Can you work these out from the model? Positions are in its coordinate system, mm. A direction names the side the tool comes from. Give positions to 0.01 mm unless a question says otherwise; leave off trailing zeros. Loops run counter-clockwise (first coordinate to the right, second up) from the corner with the lowest first, then second, coordinate; pieces in that order, holes last. Notation, with made-up numbers: (71.5, 23) -> (122.5, 23) arc R21 cw to (122.5, 37) -> close; hole circle Ø9 at (62, 67.5). An arc over 180 degrees is marked (long way). One line per question, with ' | ' between items.
from build123d import *

# Parameters (mm, degrees)
BOSS_EXTRUDE1_DEPTH      = 5
CHASSIS_WALLS1_DEPTH     = 12
CHAMFER1_SIZE            = 10
CHAMFER2_SIZE            = 10
CHAMFER3_SIZE            = 2.5
SKETCH4_R                = 1.65
CUT_EXTRUDE1_DEPTH       = 10
SKETCH5_W                = 55
SKETCH5_H                = 11
CUT_EXTRUDE2_DEPTH       = 10
SKETCH6_W                = 65
SKETCH6_H                = 5
CUT_EXTRUDE3_DEPTH       = 6
FILLET1_R                = 10
SKETCH7_W                = 42.9
SKETCH7_H                = 22
CUT_EXTRUDE4_DEPTH       = 6
SKETCH9_R                = 1.625
CUT_EXTRUDE5_DEPTH       = 6
SKETCH10_W               = 10
SKETCH10_H               = 13
SERVO_CABLE_CUTOUT_DEPTH = 10
FILLET2_R                = 2
SKETCH11_R               = 1.6
CUT_EXTRUDE6_DEPTH       = 6


with BuildPart() as part:
    # Sketch1 → Boss-Extrude1 (new body)
    with BuildSketch(Plane(origin=(0, 0, 0), x_dir=(1, 0, 0), z_dir=(0, 1, 0))):
        Polygon((-95, 35), (-65, 55), (65, 55), (95, 30), (170, 30), (170, -30), (95, -30), (65, -55), (-65, -55), (-95, -35), (-155, -35), (-155, 35), align=None)
    extrude(amount=BOSS_EXTRUDE1_DEPTH)

    # Sketch3 → Chassis-Walls1 (add)
    with BuildSketch(Plane(origin=(0, 5, 0), x_dir=(1, 0, 0), z_dir=(0, 1, 0))):
        Polygon((0, 55), (-65, 55), (-95, 35), (-92.226499019, 30.839748528), (-62.226499019, 50.839748528), (0, 50.839748528), (61.533123774, 50.839748528), (83.850910978, 32.241592525), (87.317787204, 36.401843997), (65, 55), align=None)
        Polygon((61.533123774, -50.839748528), (0, -50.839748528), (-62.226499019, -50.839748528), (-92.226499019, -30.839748528), (-95, -35), (-65, -55), (0, -55), (65, -55), (87.317787204, -36.401843997), (83.850910978, -32.241592525), align=None)
    extrude(amount=CHASSIS_WALLS1_DEPTH)

    # Chamfer1
    chamfer1_edges = [part.edges().sort_by_distance(p)[0] for p in [
        (-155, 2.5, 35),
        (-155, 2.5, -35),
    ]]
    chamfer(chamfer1_edges, length=CHAMFER1_SIZE)

    # Chamfer2
    chamfer2_edges = [part.edges().sort_by_distance(p)[0] for p in [
        (170, 2.5, -30),
        (170, 2.5, 30),
    ]]
    chamfer(chamfer2_edges, length=CHAMFER2_SIZE)

    # Chamfer3
    chamfer3_edges = [part.edges().sort_by_distance(p)[0] for p in [
        (-93.613249509, 17, -32.919874264),
        (85.584349091, 17, -34.321718261),
        (-93.613249509, 17, 32.919874264),
        (85.584349091, 17, 34.321718261),
    ]]
    chamfer(chamfer3_edges, length=CHAMFER3_SIZE)

    # Sketch4 → Cut-Extrude1 (cut)
    with BuildSketch(Plane.XZ):
        with Locations((-147, 17)):
            Circle(SKETCH4_R)
        with Locations((-55, 17)):
            Circle(SKETCH4_R)
        with Locations((-55, -17)):
            Circle(SKETCH4_R)
        with Locations((-147, -17)):
            Circle(SKETCH4_R)
        with Locations((-25, 31)):
            Circle(SKETCH4_R)
        with Locations((60, 31)):
            Circle(SKETCH4_R)
        with Locations((60, -31)):
            Circle(SKETCH4_R)
        with Locations((-25, -31)):
            Circle(SKETCH4_R)
    extrude(amount=-CUT_EXTRUDE1_DEPTH, mode=Mode.SUBTRACT)

    # Sketch5 → Cut-Extrude2 (cut)
    with BuildSketch(Plane(origin=(0, 5, 0), x_dir=(1, 0, 0), z_dir=(0, 1, 0))):
        with Locations((-127.5, -29.5)):
            Rectangle(SKETCH5_W, SKETCH5_H)
    extrude(amount=-CUT_EXTRUDE2_DEPTH, mode=Mode.SUBTRACT)

    # Sketch6 → Cut-Extrude3 (cut, through all)
    with BuildSketch(Plane(origin=(0, 5, 0), x_dir=(1, 0, 0), z_dir=(0, 1, 0))):
        with Locations((17.5, 22.5)):
            Rectangle(SKETCH6_W, SKETCH6_H)
        with Locations((17.5, -22.5)):
            Rectangle(SKETCH6_W, SKETCH6_H)
    extrude(amount=-CUT_EXTRUDE3_DEPTH, mode=Mode.SUBTRACT)

    # Fillet1
    fillet1_edges = [part.edges().sort_by_distance(p)[0] for p in [
        (-100, 2.5, 24),
    ]]
    fillet(fillet1_edges, radius=FILLET1_R)

    # Sketch7 → Cut-Extrude4 (cut, through all)
    with BuildSketch(Plane(origin=(0, 5, 0), x_dir=(1, 0, 0), z_dir=(0, 1, 0))):
        with Locations((141.25, 0)):
            Rectangle(SKETCH7_W, SKETCH7_H)
    extrude(amount=-CUT_EXTRUDE4_DEPTH, mode=Mode.SUBTRACT)

    # Sketch9 → Cut-Extrude5 (cut, through all)
    with BuildSketch(Plane(origin=(0, 5, 0), x_dir=(1, 0, 0), z_dir=(0, 1, 0))):
        with Locations((117, -19)):
            Circle(SKETCH9_R)
        with Locations((145, -19)):
            Circle(SKETCH9_R)
        with Locations((162, -17)):
            Circle(SKETCH9_R)
    cut_extrude5 = extrude(amount=-CUT_EXTRUDE5_DEPTH, mode=Mode.SUBTRACT)

    # Mirror1: Cut-Extrude5 across plane
    add(cut_extrude5.mirror(Plane.XY), mode=Mode.SUBTRACT)

    # Sketch10 → Servo-Cable-Cutout (cut)
    with BuildSketch(Plane(origin=(0, 5, 0), x_dir=(1, 0, 0), z_dir=(0, 1, 0))):
        with Locations((114.8, 0)):
            Rectangle(SKETCH10_W, SKETCH10_H)
    extrude(amount=-SERVO_CABLE_CUTOUT_DEPTH, mode=Mode.SUBTRACT)

    # Fillet2
    fillet2_edges = [part.edges().sort_by_distance(p)[0] for p in [
        (119.8, 2.5, -6.5),
        (119.8, 2.5, 6.5),
        (109.8, 2.5, 6.5),
        (109.8, 2.5, -6.5),
    ]]
    fillet(fillet2_edges, radius=FILLET2_R)

    # Sketch11 → Cut-Extrude6 (cut, through all)
    with BuildSketch(Plane(origin=(0, 5, 0), x_dir=(1, 0, 0), z_dir=(0, 1, 0))):
        with Locations((-137.6, 0)):
            Circle(SKETCH11_R)
        with Locations((-74.8, 0)):
            Circle(SKETCH11_R)
        with Locations((-64.8, 31)):
            Circle(SKETCH11_R)
        with Locations((-64.8, -31)):
            Circle(SKETCH11_R)
    extrude(amount=-CUT_EXTRUDE6_DEPTH, mode=Mode.SUBTRACT)


solid = part.part
Q1. If we section it at C-C (z = -45): Write out the boundary of the cut face in (x, y).
Entries:
outline: (-80, 0) -> (77, 0) -> (77, 17) -> (68.54, 17) -> (68.54, 5) -> (-70.99, 5) -> (-70.99, 17) -> (-80, 17) -> close
Q2. If I drill on probe 1 along Z at (x, y) = (117, 3.75) (3 decimals); probe 2 along Z at (x, y) = (-25, 1.5); probe 3 along Z at (x, y) = (61.5, 9), over which ranges is the centre line in solid material (lowest first)? Write a range as from..to.
Entries:
probe 1: -30..-20.625, -17.375..-6.5, 6.5..17.375, 20.625..30 | probe 2: -55..-32.65, -29.35..29.35, 32.65..55 | probe 3: -55..-50.84, 50.84..55
Q3. If we section it at D-D (x = -81): Write out the boundary of the cut face in (y, z), plus the area to 3 significant figures.
Entries:
outline: (0, -44.33) -> (17, -44.33) -> (17, -38.32) -> (5, -38.32) -> (5, 38.32) -> (17, 38.32) -> (17, 44.33) -> (0, 44.33) -> close | area: 588 mm²
Q4. If we mould it in two halves opening along X, with no side actions, what happens to faces 1 (the face through (1, 8, -55)), 2 (the face through (-77.016, 10.916, 40.98)), 3 (the face through (-102.85, 2.46, 27.01))? For each: pulls with the +X half, pulls with the -X half, needs draft (parallel to the pull), parting line crosses it, or undercut.
Entries:
face 1: needs draft | face 2: undercut | face 3: pulls with the -X half
Q5. For pin 1 Ø1.5 at (x, y) = (142, 3.5) entering from +Z; pin 2 Ø0.5 at (y, z) = (2.5, 34.5) entering from -X; pin 3 Ø1.5 at (x, y) = (128, 5.5) entering from -Z, each with a flat end and sliding along its axis, tell me the tip position at first contact or that it passes through.
Entries:
pin 1: z = 30 | pin 2: x = -100 | pin 3: z = -30
Q6. On a 3-axis mill with a long thin cutter (end or side, diameter ignored), from which of +Z, -Z, +X, -X, +Y, -Y can I reach the whole of each face in a straight line? I mean faces 4 (the face through (-1, 11, -50.84)), 5 (the face through (-4, 17, 52)), 6 (the face through (84.662, 15.733, 35.14)). Say none if no direction works.
Entries:
face 4: +Y | face 5: +Z, -Z, +X, -X, +Y | face 6: +X, +Y
Q7. If we section it at A-A (x = 0.5): Write out the boundary of the cut face in (y, z), plus the area to 3 significant figures.
Entries:
outline: (0, -55) -> (17, -55) -> (17, -50.84) -> (5, -50.84) -> (5, -25) -> (0, -25) -> close; (0, -20) -> (5, -20) -> (5, 20) -> (0, 20) -> close; (0, 25) -> (5, 25) -> (5, 50.84) -> (17, 50.84) -> (17, 55) -> (0, 55) -> close | area: 600 mm²
Q8. If we section it at B-B (x = -46.5): Write out the boundary of the cut face in (y, z).
Entries:
outline: (0, -55) -> (17, -55) -> (17, -50.84) -> (5, -50.84) -> (5, 50.84) -> (17, 50.84) -> (17, 55) -> (0, 55) -> close
